```python
from build123d import *

# Parameters (mm, degrees)
SKETCH1_R           = 6
BOSS_EXTRUDE1_DEPTH = 1
SKETCH2_R           = 3.5
BOSS_EXTRUDE2_DEPTH = 11
SKETCH3_R           = 6
BOSS_EXTRUDE3_DEPTH = 2
SKETCH4_R           = 6
BOSS_EXTRUDE4_DEPTH = 4
SKETCH5_R           = 2.5
CUT_EXTRUDE1_DEPTH  = 19
SKETCH6_R           = 2
CUT_EXTRUDE2_DEPTH  = 7
CIRPATTERN1_COUNT   = 2
CIRPATTERN1_ANGLE   = 90


with BuildPart() as part:
    # Sketch1 → Boss-Extrude1 (new body)
    with BuildSketch(Plane(origin=(0, 0, 0), x_dir=(1, 0, 0), z_dir=(0, 1, 0))):
        Circle(SKETCH1_R)
    extrude(amount=BOSS_EXTRUDE1_DEPTH)

    # Sketch2 → Boss-Extrude2 (add)
    with BuildSketch(Plane(origin=(0, 1, 0), x_dir=(1, 0, 0), z_dir=(0, 1, 0))):
        Circle(SKETCH2_R)
    extrude(amount=BOSS_EXTRUDE2_DEPTH)

    # Sketch3 → Boss-Extrude3 (add)
    with BuildSketch(Plane(origin=(0, 12, 0), x_dir=(1, 0, 0), z_dir=(0, 1, 0))):
        Circle(SKETCH3_R)
    extrude(amount=BOSS_EXTRUDE3_DEPTH)

    # Sketch4 → Boss-Extrude4 (add)
    with BuildSketch(Plane(origin=(0, 14, 0), x_dir=(1, 0, 0), z_dir=(0, 1, 0))):
        Circle(SKETCH4_R)
    extrude(amount=BOSS_EXTRUDE4_DEPTH)

    # Sketch5 → Cut-Extrude1 (cut, through all)
    with BuildSketch(Plane(origin=(0, 18, 0), x_dir=(1, 0, 0), z_dir=(0, 1, 0))):
        Circle(SKETCH5_R)
    extrude(amount=-CUT_EXTRUDE1_DEPTH, mode=Mode.SUBTRACT)

    # Sketch6 → Cut-Extrude2 (cut, through all)
    with BuildSketch(Plane.XY):
        with Locations((0, 14.5)):
            Circle(SKETCH6_R)
    cut_extrude2 = extrude(amount=-CUT_EXTRUDE2_DEPTH, mode=Mode.SUBTRACT)

    # CirPattern1: Cut-Extrude2 ×2 about axis
    cirpattern1_axis = Axis((0, 14, 0), (0, -1, 0))
    for i in range(1, CIRPATTERN1_COUNT):
        add(cut_extrude2.rotate(cirpattern1_axis, i * CIRPATTERN1_ANGLE / (CIRPATTERN1_COUNT - 1)), mode=Mode.SUBTRACT)


solid = part.part
```
Here's how the part is built. I have some questions about the finished solid (model axes, mm). A direction names the side the tool comes from. Coordinates: 2 decimals unless noted, no trailing zeros. Loops run counter-clockwise (first coordinate to the right, second up) from the corner with the lowest first, then second, coordinate; pieces in that order, holes last. Notation, with made-up numbers: (19, 88.25) -> (69, 88.25) arc R34 cw to (69, 126.25) -> close; hole circle Ø1 at (-31, 26.25). An arc over 180 degrees is marked (long way). Return JSON: item names as keys, results as strings.
1) Will these pins go through, and if not, where does the flat tip stop? pin 1 (5 mm diameter, centred on x = 3, y = 8.5, fed in from +Z); pin 2 (2 mm diameter, centred on y = 11.5, z = 4, fed in from -X); pin 3 (4 mm diameter, centred on x = 0, z = 0, fed in from +Y); pin 4 (2.5 mm diameter, centred on y = 14.5, z = 0, fed in from +X).
Results below:
{"pin 1": "z = 3.46", "pin 2": "x = -5.12", "pin 3": "through", "pin 4": "x = -2.17"}
2) Thinking about a two-plate mould opening in X: for faces 1 (the face through (3, 12, 3)), 2 (the face through (-2, 9.1, 1.5)), 3 (the face through (3.233, 6.423, 1.341)), which applies, +X half, -X half, draft (parallel to the pull), parting line (faces both ways), or undercut?
Results below:
{"face 1": "draft", "face 2": "undercut", "face 3": "parting line"}
3) For faces 4 (the face through (3.718, 15.101, 1.908)), 5 (the face through (3, 1, 3)), 6 (the face through (-1.998, 14.588, -3.72)), 7 (the face through (3, 18, 0)), which set-ups out of +Z, -Z, +X, -X, +Y, -Y let a thin tool reach every point of the face, with its end or its side?
Results below:
{"face 4": "+X", "face 5": "none", "face 6": "-Z", "face 7": "+Z, -Z, +X, -X, +Y"}
4) If we section it at B-B, the plane y = 15.75: Write out the boundary of the cut face in (x, z), then the cut area to 3 significant figures.
Results below:
{"outline": "(-1.56, -5.79) -> (-1.56, -1.95) arc R2.5 cw (long way) to (1.95, 1.56) -> (5.79, 1.56) arc R6 ccw (long way) to start; (1.56, -5.79) arc R6 ccw to (5.79, -1.56) -> (1.95, -1.56) arc R2.5 cw to (1.56, -1.95) -> close", "area": "70.9 mm²"}
5) I need wall thicknesses on line 1 (Y direction, x = 4.15, z = 0); line 2 (X direction, y = 10, z = 0). Which ranges of each line are inside material? Lowest first, please. Write a range as from..to.
Results below:
{"line 1": "0..1, 12..12.5, 16.5..18", "line 2": "-3.5..-2.5, 2.5..3.5"}
6) If we section it at D-D, the plane x = 0: Write out the boundary of the cut face in (y, z).
Results below:
{"outline": "(0, -6) -> (1, -6) -> (1, -3.5) -> (12, -3.5) -> (12, -6) -> (12.5, -6) -> (12.5, -2.5) -> (0, -2.5) -> close; (0, 2.5) -> (18, 2.5) -> (18, 6) -> (12, 6) -> (12, 3.5) -> (1, 3.5) -> (1, 6) -> (0, 6) -> close; (16.5, -6) -> (18, -6) -> (18, -2.5) -> (16.5, -2.5) -> close"}
7) If we section it at C-C, the plane z = 0: Write out the boundary of the cut face in (x, y).
Results below:
{"outline": "(-6, 0) -> (-2.5, 0) -> (-2.5, 18) -> (-6, 18) -> (-6, 12) -> (-3.5, 12) -> (-3.5, 1) -> (-6, 1) -> close; (2.5, 0) -> (6, 0) -> (6, 1) -> (3.5, 1) -> (3.5, 12) -> (6, 12) -> (6, 12.5) -> (2.5, 12.5) -> close; (2.5, 16.5) -> (6, 16.5) -> (6, 18) -> (2.5, 18) -> close"}
8) If we section it at A-A, the plane x = 4.75: Write out the boundary of the cut face in (y, z), then the cut area to 3 significant figures.
Results below:
{"outline": "(0, -3.67) -> (1, -3.67) -> (1, 3.67) -> (0, 3.67) -> close; (12, -3.67) -> (18, -3.67) -> (18, 3.67) -> (12, 3.67) -> close; hole circle Ø4 at (14.5, 0)", "area": "38.8 mm²"}
